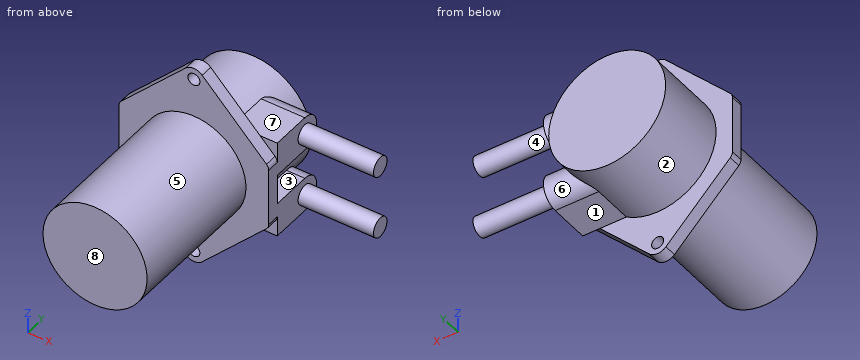
Autodesk Inventor part; units mm, degrees
ref_plane "YZ Plane" through (0, 0, 0) normal (1, 0, 0) x (0, 1, 0)
ref_plane "XZ Plane" through (0, 0, 0) normal (0, 1, 0) x (-1, 0, 0)
ref_plane "XY Plane" through (0, 0, 0) normal (0, 0, 1) x (1, 0, 0)
sketch "Sketch1" plane through (0, 0, 0) normal (0, 1, 0) x (-1, 0, 0)
  circle A0 centre (0, 0) radius 13.8
  dimension "d0" = 27.6
extrude "Extrusion1" add sketch "Sketch1" along normal blind 38.2
sketch "Sketch2" plane through (0, 38.2, 0) normal (0, 1, 0) x (1, 0, 0)
  line L0 (-19.85, -8.5) -> (19.85, -8.5) construction
  line L1 (19.85, -7.6776) -> (19.85, 7.6776)
  line L2 (19.85, 8.5) -> (-19.85, 8.5) construction
  line L3 (-19.85, 7.6776) -> (-19.85, -7.6776)
  line L4 (-19.2715, -9.0845) -> (-2.2034, -26.3306)
  line L5 (-2.2034, -26.3306) -> (2.2034, -26.3306) construction
  line L6 (2.2034, -26.3306) -> (19.2715, -9.0845)
  arc A0 (-2.2034, -26.3306) -> (2.2034, -26.3306) centre (0, -24.15) ccw
  circle A1 centre (0, -24.15) radius 1.6
  line L7 (-19.85, 0) -> (19.85, 0) construction
  line L8 (-19.2715, 9.0845) -> (-2.2034, 26.3306)
  line L9 (2.2034, 26.3306) -> (19.2715, 9.0845)
  arc A2 (2.2034, 26.3306) -> (-2.2034, 26.3306) centre (0, 24.15) ccw
  circle A3 centre (0, 24.15) radius 1.6
  arc A4 (-19.85, -7.6776) -> (-19.2715, -9.0845) centre (-17.85, -7.6776) ccw
  arc A5 (-19.2715, 9.0845) -> (-19.85, 7.6776) centre (-17.85, 7.6776) ccw
  arc A6 (19.85, 7.6776) -> (19.2715, 9.0845) centre (17.85, 7.6776) ccw
  arc A7 (19.2715, -9.0845) -> (19.85, -7.6776) centre (17.85, -7.6776) ccw
  point P0 (0, 0)
  point P1 (0, 8.5)
  point P2 (0, -27.25)
  dimension "d3" = 39.7
  dimension "d4" = 17
  dimension "d6" = 3.2
  dimension "d7" = 1.5
  dimension "d8" = 27.25
  dimension "d9" = 2
extrude "Extrusion2" add sketch "Sketch2" along normal blind 3.3
sketch "Sketch3" plane through (0, 41.5, 0) normal (0, 1, 0) x (1, 0, 0)
  circle A0 centre (0, 0) radius 13.8 construction
  circle A1 centre (0, 0) radius 15.5
  dimension "d12" = 31
extrude "Extrusion3" add sketch "Sketch3" along normal blind 19.5
sketch "Sketch4" plane through (19.85, 38.2, 7.6776) normal (1, 0, 0) x (0, 0, -1)
  line L0 (23.1776, 22.8) -> (-7.8224, 22.8)
  line L1 (-7.8224, 3.3) -> (23.1776, 3.3) construction
  line L2 (-7.8224, 3.3) -> (-7.8224, 22.8)
  line L3 (23.1776, 3.3) -> (23.1776, 22.8)
  line L4 (3.6776, 18.5) -> (11.6776, 18.5)
  line L5 (11.6776, 18.5) -> (11.6776, 3.3)
  line L6 (11.6776, 3.3) -> (3.6776, 3.3)
  line L7 (3.6776, 3.3) -> (3.6776, 18.5)
  line L8 (0, 3.3) -> (15.3553, 3.3)
  line L9 (3.6776, 18.5) -> (-5.4224, 18.5)
  line L10 (-5.4224, 18.5) -> (-5.4224, 3.3)
  line L11 (-5.4224, 3.3) -> (3.6776, 3.3)
  line L12 (3.6776, 3.3) -> (3.6776, 18.5)
  line L13 (7.6776, 3.3) -> (7.6776, 18.5) construction
  arc A0 (3.6776, 13.95) -> (-5.4224, 13.95) centre (-0.8724, 13.95) ccw
  line L14 (20.7776, 18.5) -> (20.7776, 3.3)
  line L15 (20.7776, 3.3) -> (11.6776, 3.3)
  arc A1 (20.7776, 13.95) -> (11.6776, 13.95) centre (16.2276, 13.95) ccw
  point P0 (7.6776, -38.2)
  point P1 (11.6776, 13.95)
  point P2 (3.6776, 13.95)
  dimension "d15" = 8
  dimension "d16" = 15.2
  dimension "d17" = 9.1
extrude "Extrusion4" add sketch "Sketch4" against normal up to surface contours L7 L8 L11 L10 A0 | A1 L14 L15 L8 L5
sketch "Sketch5" plane through (19.85, 38.2, 7.6776) normal (1, 0, 0) x (0, 0, -1)
  arc A0 (3.6776, 13.95) -> (-5.4224, 13.95) centre (-0.8724, 13.95) ccw
  arc A1 (20.7776, 13.95) -> (11.6776, 13.95) centre (16.2276, 13.95) ccw
  circle A2 centre (-0.8724, 13.95) radius 2.6
  circle A3 centre (16.2276, 13.95) radius 2.6
  point P0 (7.6776, -38.2)
  dimension "d20" = 5.2
  dimension "d21" = 5.2
extrude "Extrusion5" add sketch "Sketch5" along normal blind 20
equation "\"d18\" = d16"
properties part number "peristaltic pump"
Check sheet for the modelled part. Datum: model origin and axes. Units: mm. Face numbers are marked on the shaded views. A direction names the side the tool comes from. Round coordinates to 2 decimals unless told otherwise and drop trailing zeros. Loops run counter-clockwise (first coordinate to the right, second up) from the corner with the lowest first, then second, coordinate; pieces in that order, holes last.
1. Sectioned sample at D-D on x = 23. Record the boundary of the cut face in (y, z), and give its area (3 significant figures).
2. Scan lines: probe 1 along Z at (x, y) = (0, 39); probe 2 along Z at (x, y) = (18.5, 52.5); probe 3 along X at (y, z) = (40.1, 24.15). Record each from-to range of solid material in increasing order.
3. Sectioned sample at B-B on z = 24.15. Record the boundary of the cut face in (x, y), and give its area (3 significant figures).
4. Mould release check, pull along Z, two halves, no side actions. Record for the marked faces 6, 7 and 8: released by +Z, released by -Z, zero draft, split by the parting line, or undercut.
5. Sectioned sample at A-A on x = 0. Record the boundary of the cut face in (y, z), and give its area (3 significant figures).
6. Sectioned sample at C-C on z = 0. Record the boundary of the cut face in (x, y).
7. Gauge pin test, flat ends, axial feed: pin 1 Ø10 at (x, z) = (22.5, 9.5) entering from -Y; pin 2 Ø4 at (x, z) = (-7.5, 3) entering from -Y; pin 3 Ø2 at (x, y) = (1.5, 53) entering from +Z; pin 4 Ø5.5 at (x, y) = (16.5, 46.5) entering from +Z. Record the tip position at first contact, or that the pin passes through.
8. Set-up check for the marked faces 1, 2, 3, 4 and 5: record each of +Z, -Z, +X, -X, +Y, -Y from which the full face is reachable in a straight line by a thin tool's end or side.
Recorded:
1. outline: circle Ø5.2 at (52.15, -8.55); circle Ø5.2 at (52.15, 8.55)
1. area: 42.5 mm2
2. probe 1: z = -27.25 to -25.75, -22.55 to 22.55, 25.75 to 27.25
2. probe 2: z = -13.09 to -4.01, 4.01 to 13.09
2. probe 3: x = -4.36 to -1.6, 1.6 to 4.36
3. outline: (-4.36, 38.2) - (-1.6, 38.2) - (-1.6, 41.5) - (-4.36, 41.5) - close; (1.6, 38.2) - (4.36, 38.2) - (4.36, 41.5) - (1.6, 41.5) - close
3. area: 18.2 mm2
4. face 6: undercut
4. face 7: released by +Z
4. face 8: zero draft
5. outline: (0, -13.8) - (38.2, -13.8) - (38.2, -22.55) - (41.5, -22.55) - (41.5, -15.5) - (61, -15.5) - (61, 15.5) - (41.5, 15.5) - (41.5, 22.55) - (38.2, 22.55) - (38.2, 13.8) - (0, 13.8) - close; (38.2, -27.25) - (41.5, -27.25) - (41.5, -25.75) - (38.2, -25.75) - close; (38.2, 25.75) - (41.5, 25.75) - (41.5, 27.25) - (38.2, 27.25) - close
5. area: 1,820 mm2
6. outline: (-19.85, 38.2) - (-13.8, 38.2) - (-13.8, 0) - (13.8, 0) - (13.8, 38.2) - (19.85, 38.2) - (19.85, 41.5) - (15.5, 41.5) - (15.5, 61) - (-15.5, 61) - (-15.5, 41.5) - (-19.85, 41.5) - close
7. pin 1: stops at y = 38.2
7. pin 2: stops at y = 0
7. pin 3: stops at z = 15.49
7. pin 4: stops at z = 13.1
8. face 1: -Z, +X, +Y
8. face 2: +Y
8. face 3: +X, +Y
8. face 4: +X
8. face 5: -Y
